The listing builds one solid part. Answer for the finished solid, in the listing's coordinates (mm). A direction names the side the tool comes from. Round coordinates to 2 decimals unless told otherwise and drop trailing zeros. Write each loop counter-clockwise with the first axis right and the second up, starting at its lowest first coordinate (ties: lowest second). Pieces come first, ordered by that corner, then holes.
from build123d import *

# Parameters (mm, degrees)
F1_DEPTH    = 10
F2_T1_DEPTH = 10
F2_T3_DEPTH = 34.4948974279
F2_T5_DEPTH = 34.4948974279
F3_R        = 3
F4_R        = 1.59999


# Not quite as in the source:
# - a fillet or chamfer that OpenCascade refuses, or shapes differently, is made with other operations: its cross-section is extruded or revolved along the edge and cut away or added
# - a fillet or chamfer is up to 0.001 mm smaller than in the source, because OpenCascade refuses the exact size


with BuildPart() as f1:
    # F0 (on Top) → F1 (new body)
    with BuildSketch(Plane.XY):
        with BuildLine():
            Line((-7.7799167484, 4), (-7.7799167484, 0))
            Line((-7.7799167484, 0), (37.5679595768, 0))
            Line((37.5679595768, 0), (37.5679595768, 4))
            Line((37.5679595768, 4), (21.6996651143, 4))
            ThreePointArc((21.6996651143, 4), (13.9894641382, 7.0819259987), (9.5494964602, 14.0984888306))
            Line((9.5494964602, 14.0984888306), (15.7092516907, 30.1592148483))
            Line((15.7092516907, 30.1592148483), (14.215355652, 30.732167399))
            Line((14.215355652, 30.732167399), (4.170825278, 4.5424172749))
            Line((4.170825278, 4.5424172749), (2.2100867272, 5.2944174977))
            Line((2.2100867272, 5.2944174977), (12.2367563651, 31.4375981759))
            Line((12.2367563651, 31.4375981759), (10.7428603263, 32.0105507266))
            Line((10.7428603263, 32.0105507266), (0, 4))
            Line((0, 4), (-7.7799167484, 4))
        make_face()
    extrude(amount=F1_DEPTH)

    # F2: fillet of radius 5 on 3 edges, made by hand

    # F2_s2 → F2_t1 (join)
    with BuildSketch(Plane.XY):
        with BuildLine():
            ThreePointArc((10.2974988853, 11.9526797446), (9.8650823787, 13.8567183835), (10.1948614585, 15.7811905013))
            Line((10.1948614585, 15.7811905013), (9.5494964602, 14.0984888306))
            ThreePointArc((9.5494964602, 14.0984888306), (9.8781857469, 13.0097891124), (10.2974988853, 11.9526797446))
        make_face()
    extrude(amount=F2_T1_DEPTH)

    # F2_s4 → F2_t3 (cut)
    with BuildSketch(Plane.XY.offset(-12.2474487139)):
        with BuildLine():
            ThreePointArc((-2.8809372628, 4), (-6.043214923, 2.8729833462), (-7.7799167484, 0))
            Line((-7.7799167484, 0), (-7.7799167484, 4))
            Line((-7.7799167484, 4), (-2.8809372628, 4))
        make_face()
    extrude(amount=F2_T3_DEPTH, mode=Mode.SUBTRACT)

    # F2_s6 → F2_t5 (cut)
    with BuildSketch(Plane.XY.offset(-12.2474487139)):
        with BuildLine():
            ThreePointArc((32.6689800913, 4), (35.8312577514, 2.8729833462), (37.5679595768, 0))
            Line((37.5679595768, 0), (37.5679595768, 4))
            Line((37.5679595768, 4), (32.6689800913, 4))
        make_face()
    extrude(amount=F2_T5_DEPTH, mode=Mode.SUBTRACT)

    # F3
    f3_edges = [f1.edges().sort_by_distance(p)[0] for p in [
        (0, 4, 5),
    ]]
    fillet(f3_edges, radius=F3_R)

    # F4 (radius 1.6 in the source; OpenCascade refuses exactly that, so slightly less here)
    f4_edges = [f1.edges().sort_by_distance(p)[0] for p in [
        (12.236756, 31.437598, 5),
        (14.215356, 30.732167, 5),
    ]]
    fillet(f4_edges, radius=F4_R)


solid = f1.part
1. Section B-B on x = 3.5 is taken. Determine the outline of the cut face in (y, z), plus the area to 3 significant figures.
Geometry says:
outline: (0, 0) - (4.8, 0) - (4.8, 10) - (0, 10) - close; (8.66, 0) - (13.13, 0) - (13.13, 10) - (8.66, 10) - close
area: 92.7 mm2
2. Section D-D on x = 31 is taken. Determine the outline of the cut face in (y, z), plus the area to 3 significant figures.
Geometry says:
outline: (0, 0) - (4, 0) - (4, 10) - (0, 10) - close
area: 40.0 mm2
3. For a pull along X with two mould halves and no side action, classify faces 5 (the face through (9.866, 13.829, 4.93)), 6 (the face through (8.97, 17.06, 4.93)), 7 (the face through (-0.384, 4.514, 5.07)) as released by +X, released by -X, zero draft, split by the parting line, or undercut.
Geometry says:
face 5: released by +X
face 6: undercut
face 7: released by -X
4. Given pin 1 (5 mm diameter, centred on x = 25, z = 4, fed in from +Y); pin 2 (1 mm diameter, centred on y = 27.5, z = 6, fed in from +X); pin 3 (5 mm diameter, centred on y = 11, z = 8.5, fed in from -X), each flat-ended and moving along its own axis, determine where each tip first touches the part or whether it passes through.
Geometry says:
pin 1: stops at y = 4
pin 2: stops at x = 14.88
pin 3: stops at x = 1.73
5. Straight lines are drawn through the part: line 1 along Y through (x, z) = (29.5, 7.75); line 2 along X through (y, z) = (18.5, 1); line 3 along X through (y, z) = (9, 4.25). For each, find the intervals that lie inside material, in ascending order.
Geometry says:
line 1: y = 0 to 4
line 2: x = 5.56 to 7.27, 9.52 to 11.24
line 3: x = 1.92 to 3.63, 5.88 to 12.1
6. Section A-A on y = 12.5 is taken. Determine the outline of the cut face in (x, z).
Geometry says:
outline: (3.26, 0) - (4.97, 0) - (4.97, 10) - (3.26, 10) - close; (7.22, 0) - (10.09, 0) - (10.09, 10) - (7.22, 10) - close
7. A tool of negligible diameter and unlimited length cuts with its end or side. For faces 1 (the face through (14.47, 30.12, 5.07)), 2 (the face through (27, 4, 5)), 3 (the face through (12.913, 22.87, 4.93)), 4 (the face through (6.87, 17.45, 4.93)), from which of +Z, -Z, +X, -X, +Y, -Y can it reach the whole face along a straight path? Write none if from no direction.
Geometry says:
face 1: +Z, -Z, +Y
face 2: +Z, -Z, +X, +Y
face 3: +Z, -Z, +X
face 4: +Z, -Z
